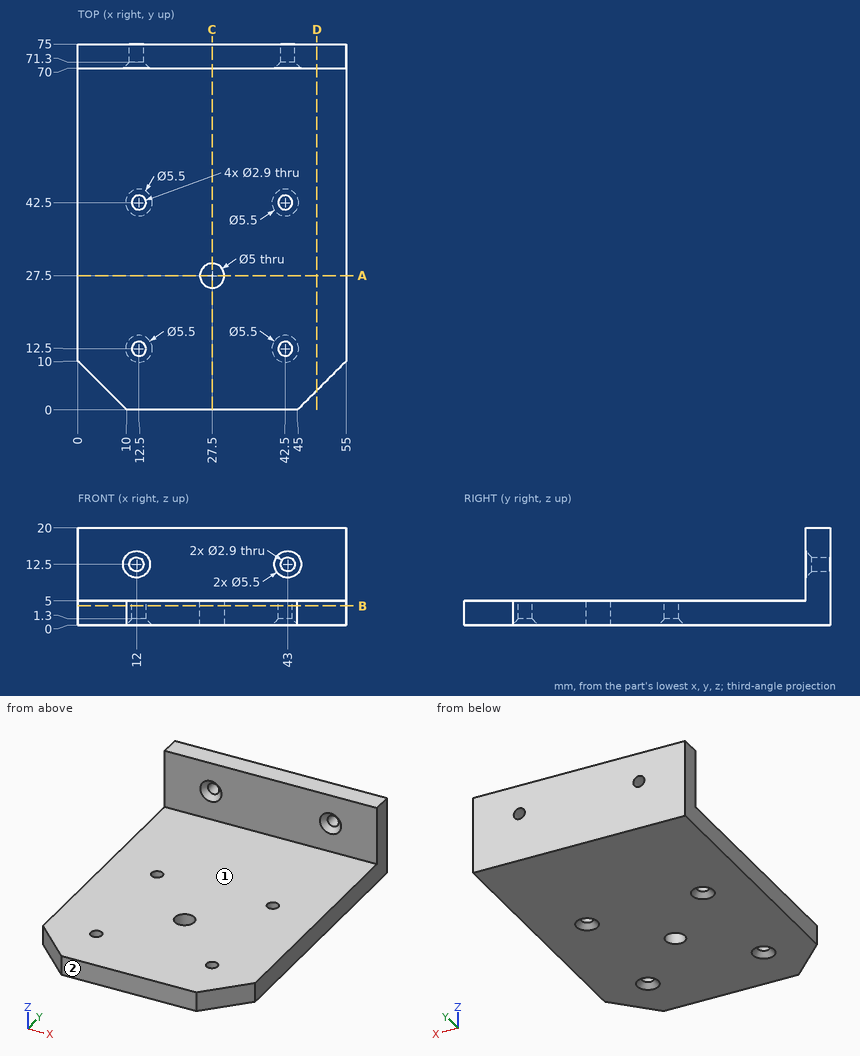
Check sheet for the drawn part. Datum: minimum x, y, z corner. Units: mm. A direction names the side the tool comes from. Give positions to 0.01 mm unless a question says otherwise; leave off trailing zeros. Order: outer loops, then holes, each group sorted by start corner. A loop starts at its lowest first (then second) coordinate and runs counter-clockwise, first axis right, second up. Notation, with made-up numbers: (-27, -3) -> (-10, -3) arc R25 ccw to (-10, 9) -> close; hole circle Ø7 at (15, -17). An arc over 180 degrees is marked (long way). Answer as CSV lines item,"result".
Q1. Scan lines: probe 1 along X at (y, z) = (42.5, 3.8); probe 2 along Y at (x, z) = (12.5, 4.2); probe 3 along X at (y, z) = (73.75, 12.5). Record each from-to range of solid material in increasing order.
Solutions:
probe 1,"x = 0 to 11.05, 13.95 to 41.05, 43.95 to 55"
probe 2,"y = 0 to 11.05, 13.95 to 41.05, 43.95 to 75"
probe 3,"x = 0 to 10.55, 13.45 to 41.55, 44.45 to 55"
Q2. Sectioned sample at C-C on x = 27.5. Record the cut outline in (y, z), plus the area to 3 significant figures.
Solutions:
outline,"(0, 0) -> (25, 0) -> (25, 5) -> (0, 5) -> close; (30, 0) -> (75, 0) -> (75, 20) -> (70, 20) -> (70, 5) -> (30, 5) -> close"
area,"425 mm²"
Q3. Depth check by flat-ended pin: pin 1 (8 mm diameter, centred on x = 45, y = 18, fed in from +Z); pin 2 (7.5 mm diameter, centred on x = 20.5, z = 15.5, fed in from -Y); pin 3 (4.5 mm diameter, centred on x = 43, z = 12.5, fed in from -Y). Enter the tip coordinate at first touch or a pass-through.
Solutions:
pin 1,"stops at z = 5"
pin 2,"stops at y = 70"
pin 3,"stops at y = 70.5"
Q4. Sectioned sample at D-D on x = 49. Record the cut outline in (y, z).
Solutions:
outline,"(4, 0) -> (75, 0) -> (75, 20) -> (70, 20) -> (70, 5) -> (4, 5) -> close"
Q5. Access from +Z, -Z, +X, -X, +Y, -Y to the whole of each face (thin tool, end or side, straight path). Record for the marked faces 1 and 2.
Solutions:
face 1,"+Z, +X, -X, -Y"
face 2,"+Z, -Z, +X, -X, -Y"
Q6. Sectioned sample at B-B on z = 4. Record the cut outline in (x, y), plus the area to 3 significant figures.
Solutions:
outline,"(0, 10) -> (10, 0) -> (45, 0) -> (55, 10) -> (55, 75) -> (0, 75) -> close; hole circle Ø2.9 at (12.5, 12.5); hole circle Ø2.9 at (12.5, 42.5); hole circle Ø5 at (27.5, 27.5); hole circle Ø2.9 at (42.5, 12.5); hole circle Ø2.9 at (42.5, 42.5)"
area,"3,980 mm²"
Q7. Sectioned sample at A-A on y = 27.5. Record the cut outline in (x, z), plus the area to 3 significant figures.
Solutions:
outline,"(0, 0) -> (25, 0) -> (25, 5) -> (0, 5) -> close; (30, 0) -> (55, 0) -> (55, 5) -> (30, 5) -> close"
area,"250 mm²"
